```python
from build123d import *

# Parameters (mm, degrees)
BOSS_EXTRUDE1_DEPTH = 20
SKETCH2_W           = 9
SKETCH2_H           = 25
BOSS_EXTRUDE2_DEPTH = 1
BOSS_EXTRUDE2_TAPER = 45
SKETCH3_W           = 25
SKETCH3_H           = 9
BOSS_EXTRUDE3_DEPTH = 1
BOSS_EXTRUDE3_TAPER = 45
CUT_EXTRUDE3_DEPTH  = 3.5
SKETCH9_W           = 10
SKETCH9_H           = 8.5
CUT_EXTRUDE4_DEPTH  = 7
CHAMFER3_START      = 7.5
CHAMFER3_DEPTH      = 5
CHAMFER3_START_2    = 5
CHAMFER3_2_DEPTH    = 10
CHAMFER3_START_3    = 0.671572875
CHAMFER3_3_DEPTH    = 2.5
CUT_EXTRUDE5_REACH  = 43.857
SKETCH4_R           = 2.6
CUT_EXTRUDE6_REACH  = 43.243
SKETCH5_R           = 2.6


with BuildPart() as part:
    # Sketch1 → Boss-Extrude1 (new body)
    with BuildSketch(Plane.XY):
        Polygon((0, 0), (0, 4), (21, 25), (25, 25), (25, 0), align=None)
    extrude(amount=BOSS_EXTRUDE1_DEPTH)

    # Sketch2 → Boss-Extrude2 (add)
    with BuildSketch(Plane(origin=(25, 0, 0), x_dir=(0, 0, -1), z_dir=(1, 0, 0))):
        with Locations((-10, 12.5)):
            Rectangle(SKETCH2_W, SKETCH2_H)
    extrude(amount=BOSS_EXTRUDE2_DEPTH, taper=BOSS_EXTRUDE2_TAPER)

    # Sketch3 → Boss-Extrude3 (add)
    with BuildSketch(Plane.XZ):
        with Locations((12.5, 10)):
            Rectangle(SKETCH3_W, SKETCH3_H)
    extrude(amount=BOSS_EXTRUDE3_DEPTH, taper=BOSS_EXTRUDE3_TAPER)

    # Sketch7 → Cut-Extrude3 (cut)
    with BuildSketch(Plane(origin=(-2, 2, 0), x_dir=(0, 0, 1), z_dir=(-0.7071067811865464, 0.7071067811865487, 0))):
        with BuildLine():
            Line((7.5, 29.026911935), (12.5, 29.026911935))
            ThreePointArc((12.5, 29.026911935), (14.267766953, 28.294678888), (15, 26.526911935))
            Line((15, 26.526911935), (15, 8.826911935))
            ThreePointArc((15, 8.826911935), (14.267766953, 7.059144982), (12.5, 6.326911935))
            Line((12.5, 6.326911935), (7.5, 6.326911935))
            ThreePointArc((7.5, 6.326911935), (5.732233047, 7.059144982), (5, 8.826911935))
            Line((5, 8.826911935), (5, 26.526911935))
            ThreePointArc((5, 26.526911935), (5.732233047, 28.294678888), (7.5, 29.026911935))
        make_face()
    extrude(amount=-CUT_EXTRUDE3_DEPTH, mode=Mode.SUBTRACT)

    # Sketch9 → Cut-Extrude4 (cut)
    with BuildSketch(Plane(origin=(0.474873734, -0.474873734, 0), x_dir=(0, 0, 1), z_dir=(-0.7071067811865464, 0.7071067811865487, 0))):
        with Locations((10, 17.676911935)):
            Rectangle(SKETCH9_W, SKETCH9_H)
    extrude(amount=-CUT_EXTRUDE4_DEPTH, mode=Mode.SUBTRACT)

    # Chamfer3: read off the stored shape, not the designer's step
    # Chamfer3 outline → Chamfer3 (cut)
    with BuildSketch(Plane.XY.offset(CHAMFER3_START)):
        Polygon((15.979541854, 15.029794385), (20.929289322, 10.080046917), (21, 10.150757595), (21, 20.050252532), align=None)
        Polygon((4.948676067, 3.998928599), (14.848171004, 3.998928599), (14.918881682, 4.069639277), (9.969134213, 9.019386745), align=None)
    extrude(amount=CHAMFER3_DEPTH, mode=Mode.SUBTRACT)

    # Chamfer3 2 outline → Chamfer3 2 (cut)
    with BuildSketch(Plane.XY.offset(CHAMFER3_START_2)):
        Polygon((15.979541854, 15.029794385), (20.929289322, 10.080046917), (21, 10.150757595), (21, 20.050252532), align=None)
        Polygon((4.948676067, 3.998928599), (14.848171004, 3.998928599), (14.918881682, 4.069639277), (9.969134213, 9.019386745), align=None)
    extrude(amount=CHAMFER3_2_DEPTH, mode=Mode.SUBTRACT)

    # Chamfer3 3 outline → Chamfer3 3 (add)
    with BuildSketch(Plane(origin=(0, 0, 0), x_dir=(0.707106781186549, 0.707106781186546, 0), z_dir=(0.707106781186546, -0.707106781186549, 0)).offset(CHAMFER3_START_3)):
        with BuildLine():
            Line((6.326911935, 5.000000001), (8.826911935, 5))
            ThreePointArc((8.826911935, 5), (7.059144982, 5.732233047), (6.326911935, 7.5))
            Line((6.326911935, 7.5), (6.326911935, 5.000000001))
        make_face()
        with BuildLine():
            ThreePointArc((29.026911935, 7.5), (28.294678888, 5.732233047), (26.526911935, 5))
            Line((26.526911935, 5), (29.026911935, 5.000000001))
            Line((29.026911935, 5.000000001), (29.026911935, 7.5))
        make_face()
        with BuildLine():
            Line((6.326911935, 14.999999999), (6.326911935, 12.5))
            ThreePointArc((6.326911935, 12.5), (7.059144982, 14.267766953), (8.826911935, 15))
            Line((8.826911935, 15), (6.326911935, 14.999999999))
        make_face()
        with BuildLine():
            ThreePointArc((26.526911935, 15), (28.294678888, 14.267766953), (29.026911935, 12.5))
            Line((29.026911935, 12.5), (29.026911935, 14.999999999))
            Line((29.026911935, 14.999999999), (26.526911935, 15))
        make_face()
    extrude(amount=CHAMFER3_3_DEPTH)

    # Sketch4 → Cut-Extrude5 (cut, up to next)
    with BuildSketch(Plane.XZ.offset(1), mode=Mode.PRIVATE) as cut_extrude5_sk1:
        with Locations(Location((9, 10, 0), (0, 0, 270))):
            Circle(SKETCH4_R)
    cut_extrude5_tool1 = extrude(cut_extrude5_sk1.sketch, amount=-CUT_EXTRUDE5_REACH, mode=Mode.PRIVATE) & part.part
    add(cut_extrude5_tool1.solids().sort_by_distance((9, -1, 10))[0], mode=Mode.SUBTRACT)

    # Sketch5 → Cut-Extrude6 (cut, up to next)
    with BuildSketch(Plane(origin=(26, 0, 0), x_dir=(0, 0, -1), z_dir=(1, 0, 0)), mode=Mode.PRIVATE) as cut_extrude6_sk1:
        with Locations(Location((-10, 15, 0), (0, 0, 90))):
            Circle(SKETCH5_R)
    cut_extrude6_tool1 = extrude(cut_extrude6_sk1.sketch, amount=-CUT_EXTRUDE6_REACH, mode=Mode.PRIVATE) & part.part
    add(cut_extrude6_tool1.solids().sort_by_distance((26, 15, 10))[0], mode=Mode.SUBTRACT)


solid = part.part
```
The model under review builds one solid part; all positions refer to its coordinate system, in mm. A direction names the side the tool comes from. Round coordinates to 2 decimals unless told otherwise and drop trailing zeros. Write each loop counter-clockwise with the first axis right and the second up, starting at its lowest first coordinate (ties: lowest second). Pieces come first, ordered by that corner, then holes. Notation, with made-up numbers: (44.5, -36.5) - (87.5, -36.5) arc R13 cw to (87.5, -29.5) - close; hole circle Ø6 at (9.5, -8). An arc over 180 degrees is marked (long way). Use one line per item in the form item = value.
Q1. Insertion check: pin 1 Ø6 at (y, z) = (15.5, 3) entering from +X; pin 2 Ø3 at (x, z) = (11, 12) entering from +Y; pin 3 Ø3 at (y, z) = (15, 10) entering from -X; pin 4 Ø1.6 at (x, z) = (10, 17) entering from -Y. Each pin has a flat end and moves straight along its axis. Give the tip position at first contact, or say it passes through.
Answer key:
pin_1 = 25.5
pin_2 = 4
pin_3 = through
pin_4 = 0
Q2. For line 1 (Z direction, x = 23.9, y = 15); line 2 (X direction, y = 2.65, z = 10); line 3 (Y direction, x = 22.25, z = 11), list the stretches that pass through material, from the lowest coordinate up. Write a range as [from, to].
Answer key:
line_1 = [0, 7.4], [12.6, 20]
line_2 = [0, 6.4], [11.6, 26]
line_3 = [-1, 12.6], [17.4, 25]
Q3. Tool access review of faces 4 (the cylindrical face through (19.38, 20.14, 5.44)), 5 (the flat face through (25, 13, 3)), 6 (the flat face through (14, 11, 5)), 7 (the flat face through (3.694, 5.254, 10.035)): name each direction out of +Z, -Z, +X, -X, +Y, -Y from which nothing blocks a thin tool from reaching the whole face with its end or side.
Answer key:
face_4 = -X
face_5 = -Z, +X, +Y, -Y
face_6 = none
face_7 = +Y
Q4. Consider section B-B (z = 10). State how many separate pieces and enclosed holes the cut face has, and give its area (3 significant figures).
Answer key:
separate_pieces = 3
enclosed_holes = 0
area = 211 mm2
Q5. Consider section A-A (z = 1.5). State the section outline as (x, y) points.
Answer key:
outline = (0, 0) - (25, 0) - (25, 25) - (21, 25) - (0, 4) - close
Q6. Draft analysis for pull direction Z (two halves, no side actions). For faces 1 (the flat face through (14, 11, 15)), 2 (the flat face through (23, 25, 10)), 3 (the flat face through (15, 10, 20)), state which applies: +Z half, -Z half, draft (parallel to the pull), parting line (faces both ways), or undercut.
Answer key:
face_1 = undercut
face_2 = draft
face_3 = +Z half
